```python
from build123d import *

# Parameters (mm, degrees)
SKETCH4_R           = 3.58775
BOSS_EXTRUDE1_DEPTH = 9.525


with BuildPart() as part:
    # Sketch3 → Revolve1 (revolve)
    with BuildSketch(Plane(origin=(0, 0, 0), x_dir=(0, 0, -1), z_dir=(1, 0, 0))):
        Polygon((-4.7498, 2.413), (-4.7498, 0), (9.525, 0), (9.525, 2.413), (1.44065625, 2.413), (1.143, 1.897444252), (0, 1.897444252), (0, 4.7625), (-9.525, 4.7625), (-9.525, 2.413), align=None)
    revolve(axis=Axis((0, 0, -9.525), (0, 0, 1)))

    # Sketch4 → Boss-Extrude1 (add)
    with BuildSketch(Plane.XY.offset(9.525)):
        Polygon((-4.7625, 2.749630657), (-4.7625, -2.749630657), (0, -5.499261314), (4.7625, -2.749630657), (4.7625, 2.749630657), (0, 5.499261314), align=None)
        Circle(SKETCH4_R, mode=Mode.SUBTRACT)
    extrude(amount=-BOSS_EXTRUDE1_DEPTH)


solid = part.part
```
Source: CAD feature listing. Evaluate the final solid. Frame: model axes, mm. A direction names the side the tool comes from. Give positions to 0.01 mm unless a question says otherwise; leave off trailing zeros. Loops run counter-clockwise (first coordinate to the right, second up) from the corner with the lowest first, then second, coordinate; pieces in that order, holes last. Notation, with made-up numbers: (9, -38.5) -> (44, -38.5) arc R30 ccw to (44, -5.5) -> close; hole circle Ø7 at (-10, 0.25). An arc over 180 degrees is marked (long way). Put each result on its own line as item: value. Start each with the question number.
1) Reachability of faces 1 (the face through (1.468, -1.915, -5.426)), 2 (the face through (4.762, 0, 5)), 3 (the face through (0, 0, 4.75)) from +Z, -Z, +X, -X, +Y, -Y: full face, straight path, thin tool, end or side. Return the list, or none.
2) Contact query for flat-ended pins moving along their axis: P1, Ø2, axis at x = -1, z = -5.5, coming from the -Y side; P2, Ø1.4, axis at x = 1, y = -0.5, coming from the +Z side; P3, Ø2, axis at x = 3, z = -5.5, coming from the +Y side. Output: stop coordinate, or through.
3) Draft query along Z for faces 4 (the face through (-1.1, -2.4, 9.525)), 5 (the face through (1.15, -1.51, -0.56)), 6 (the face through (1.468, -1.915, 7.104)). Return one class per face: released by +Z, released by -Z, zero draft, split by the parting line, or undercut.
4) Cut plane A-A (z = 5.25). Return loops of the section in (x, y).
5) Cut plane C-C (z = 2.25). Return loops of the section in (x, y).
6) Cut plane B-B (y = 0). Return loops of the section in (x, z) (1 decimal).
7) Material intervals for probe 1 along X at (y, z) = (0, 7.9); probe 2 along Z at (x, y) = (1.5, 0) (3 decimals); probe 3 along Z at (x, y) = (-0.75, -3.75) (3 decimals), sorted ascending.
8) Cut plane D-D (x = 3.25). Return loops of the section in (y, z) (3 decimals).
Results are:
1. face 1: -Z
1. face 2: +Z, -Z, +X, +Y, -Y
1. face 3: +Z
2. P1: stops at y = -2.41
2. P2: stops at z = 4.75
2. P3: stops at y = 1.35
3. face 4: released by +Z
3. face 5: undercut
3. face 6: zero draft
4. outline: (-4.76, -2.75) -> (0, -5.5) -> (4.76, -2.75) -> (4.76, 2.75) -> (0, 5.5) -> (-4.76, 2.75) -> close; hole circle Ø4.83 at (0, 0)
5. outline: (-4.76, -2.75) -> (0, -5.5) -> (4.76, -2.75) -> (4.76, 2.75) -> (0, 5.5) -> (-4.76, 2.75) -> close
6. outline: (-4.8, 0) -> (-1.9, 0) -> (-1.9, -1.1) -> (-2.4, -1.4) -> (-2.4, -9.5) -> (2.4, -9.5) -> (2.4, -1.4) -> (1.9, -1.1) -> (1.9, 0) -> (4.8, 0) -> (4.8, 9.5) -> (2.4, 9.5) -> (2.4, 4.7) -> (-2.4, 4.7) -> (-2.4, 9.5) -> (-4.8, 9.5) -> close
7. probe 1: x = -4.76 to -2.41, 2.41 to 4.76
7. probe 2: z = -9.525 to 4.75
7. probe 3: z = 0 to 9.525
8. outline: (-3.623, 0) -> (3.623, 0) -> (3.623, 9.525) -> (-3.623, 9.525) -> close
